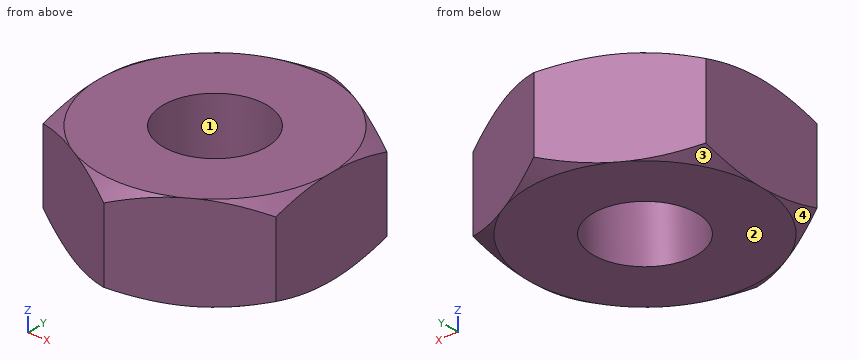
Solid Edge part; units mm, degrees
sketch "Sketch1" plane through (0, 0, 0) normal (0, 0, 1) x (1, 0, 0)
  line L0 (2.75, 1.5877) -> (0, 3.1754)
  line L1 (0, 3.1754) -> (-2.75, 1.5877)
  line L2 (-2.75, 1.5877) -> (-2.75, -1.5877)
  line L3 (-2.75, -1.5877) -> (0, -3.1754)
  line L4 (0, -3.1754) -> (2.75, -1.5877)
  line L5 (2.75, -1.5877) -> (2.75, 1.5877)
extrude "Protrusion1" add sketch "Sketch1" along normal mid plane 2.25
hole "Agujero_1" at (0, 0, 1.125) direction (0, 0, -1) diameter 2.459 end up to next
sketch "Sketch2" plane through (0, 0, 0) normal (0, -1, 0) x (1, 0, 0)
  line L0 (2.75, 1.125) -> (4.6986, 0)
revolve "RevolvedCutout1" cut sketch "Sketch2" angle 360 about axis through (0, 0, 54) along (0, 0, -1) material side at (3.7493, 0, 0.6058)
mirror "Mirror1" about plane through (0, 0, 0) normal (0, 0, 1) of "RevolvedCutout1"
Geometry check sheet. Reference: the model listing, model coordinates, mm. Face numbers are marked on the shaded views. Give positions to 0.01 mm unless a question says otherwise; leave off trailing zeros. Order: outer loops, then holes, each group sorted by start corner. A loop starts at its lowest first (then second) coordinate and runs counter-clockwise, first axis right, second up. Notation, with made-up numbers: (3, 68.25) - (43, 68.25) arc R22 cw to (43, 84.25) - close; hole circle Ø6 at (86.25, -31). An arc over 180 degrees is marked (long way). Answer in a Markdown table with one row per item. Add a question column.
Q1. Gauge pin test, flat end, axial feed: pin 1 (3 mm diameter, centred on x = 1, y = -0.5, fed in from -Z) (3 decimals). Record the tip position at first contact, or that the pin passes through.
Q2. Material ranges on probe 1 along X at (y, z) = (0, -0.05); probe 2 along Y at (x, z) = (-0.55, -0.4); probe 3 along X at (y, z) = (2, -0.6), recorded low to high. Write a range as from..to.
Q3. Cross-section at A-A, the plane z = -0.5. Enter the section's corners in (x, y), then the cut area to 3 significant figures.
Q4. Mould release check, pull along Y, two halves, no side actions. Record for the marked faces 1, 2, 3 and 4: pulls with the +Y half, pulls with the -Y half, needs draft (parallel to the pull), parting line crosses it, or undercut.
Check values:
| question | item | result |
|---|---|---|
| 1 | pin 1 | stops at z = -1.125 |
| 2 | probe 1 | x = -2.75..-1.23, 1.23..2.75 |
| 2 | probe 2 | y = -2.86..-1.1, 1.1..2.86 |
| 2 | probe 3 | x = -2.04..2.04 |
| 3 | outline | (-2.75, -1.59) - (0, -3.18) - (2.75, -1.59) - (2.75, 1.59) - (0, 3.18) - (-2.75, 1.59) - close; hole circle Ø2.46 at (0, 0) |
| 3 | area | 21.4 mm^2 |
| 4 | face 1 | undercut |
| 4 | face 2 | needs draft |
| 4 | face 3 | pulls with the +Y half |
| 4 | face 4 | pulls with the -Y half |
